Source: CAD feature listing. Evaluate the final solid. Frame: model axes, mm. Face numbers are marked on the shaded views. A direction names the side the tool comes from. Coordinates: 2 decimals unless noted, no trailing zeros. Loops run counter-clockwise (first coordinate to the right, second up) from the corner with the lowest first, then second, coordinate; pieces in that order, holes last. Notation, with made-up numbers: (3.25, 11) -> (15.25, 11) arc R12 ccw to (15.25, 30) -> close; hole circle Ø7 at (37, -33.75). An arc over 180 degrees is marked (long way). Answer as a JSON object with one key per item and string values. Group by question number.
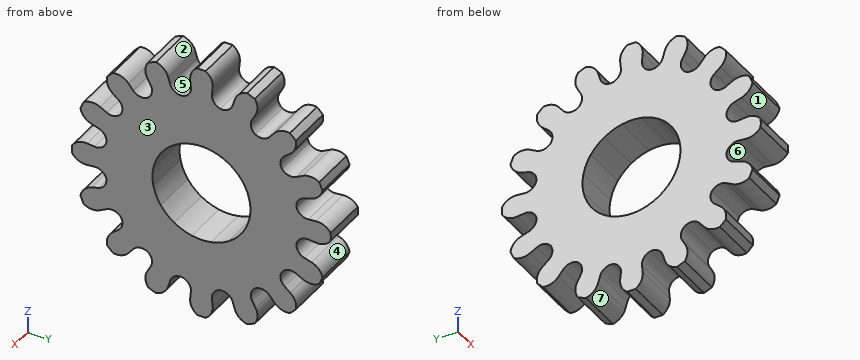
from build123d import *

# Parameters (mm, degrees)
BOSS_EXTRUDE2_DEPTH = 3.175
FILLET1_R           = 0.767540966
CIRPATTERN1_COUNT   = 16
SKETCH2_R           = 3.41
CUT_EXTRUDE1_DEPTH  = 14.117950488


with BuildPart() as part:
    # Sketch1 → Boss-Extrude2 (new body)
    with BuildSketch(Plane(origin=(0, 0, 0), x_dir=(0, 0, -1), z_dir=(1, 0, 0))):
        with BuildLine():
            Line((6.717496905, 0.661615697), (7.961477813, 0.784137123))
            ThreePointArc((7.961477813, 0.784137123), (8.546163052, 0.682503707), (8.995181287, 0.294471745))
            ThreePointArc((8.995181287, 0.294471745), (9, 0), (8.995181287, -0.294471745))
            ThreePointArc((8.995181287, -0.294471745), (8.546163052, -0.682503707), (7.961477813, -0.784137123))
            Line((7.961477813, -0.784137123), (6.717496905, -0.661615697))
            ThreePointArc((6.717496905, -0.661615697), (6.676941442, -0.990430703), (6.620300643, -1.316859674))
            Line((6.620300643, -1.316859674), (0, 0))
            Line((0, 0), (6.620300643, 1.316859674))
            ThreePointArc((6.620300643, 1.316859674), (6.676941442, 0.990430703), (6.717496905, 0.661615697))
        make_face()
    extrude(amount=BOSS_EXTRUDE2_DEPTH)

    # Fillet1
    # the kernel refuses this fillet: 0.767540966 mm, written as the material it adds along each edge
    with BuildSketch(Plane(origin=(0, 0.661615697, -6.717496905), x_dir=(0, 0.9888733768354266, 0.14875968736892464), z_dir=(1, 0, 0))) as fillet1_piece_1_section:
        with BuildLine():
            CenterArc((0.729311441, -0.766537545), FILLET1_R, 92.930055473, 84.139889054)
            Line((-0.037226104, -0.727303285), (0, 0))
            ThreePointArc((0, 0), (0.345038591, -0.008824407), (0.690077182, 0))
        make_face()
    fillet1_piece_1 = extrude(amount=3.175, mode=Mode.PRIVATE)
    fillet1_piece_1 = split(fillet1_piece_1, bisect_by=Plane(origin=(1.5875, 1.34516519, -6.762602082), z_dir=(0, -0.9807852804032304, -0.19509032201612872)), keep=Keep.TOP, mode=Mode.PRIVATE)
    add(fillet1_piece_1)
    with BuildSketch(Plane(origin=(0, -0.661615697, -6.717496905), x_dir=(0, -0.09801714032956141, -0.9951847266721968), z_dir=(1, 0, 0))) as fillet1_piece_2_section:
        with BuildLine():
            CenterArc((0.728255348, -0.767540966), FILLET1_R, 90, 84.139889054)
            ThreePointArc((-0.035274557, -0.68917503), (-0.008824407, -0.345038591), (0, 0))
            Line((0, 0), (0.728255348, 0))
        make_face()
    fillet1_piece_2 = extrude(amount=3.175, mode=Mode.PRIVATE)
    fillet1_piece_2 = split(fillet1_piece_2, bisect_by=Plane(origin=(1.5875, -1.34516519, -6.762602082), z_dir=(0, 0.9807852804032304, -0.19509032201612872)), keep=Keep.TOP, mode=Mode.PRIVATE)
    add(fillet1_piece_2)


with BuildPart() as cirpattern1_1:
    # CirPattern1: pattern copy
    add(part.part.rotate(Axis((0, 0, 0), (1, 0, 0)), 1 * 360 / CIRPATTERN1_COUNT))


with BuildPart() as cirpattern1_2:
    # CirPattern1: pattern copy
    add(part.part.rotate(Axis((0, 0, 0), (1, 0, 0)), 2 * 360 / CIRPATTERN1_COUNT))


with BuildPart() as cirpattern1_3:
    # CirPattern1: pattern copy
    add(part.part.rotate(Axis((0, 0, 0), (1, 0, 0)), 3 * 360 / CIRPATTERN1_COUNT))


with BuildPart() as cirpattern1_4:
    # CirPattern1: pattern copy
    add(part.part.rotate(Axis((0, 0, 0), (1, 0, 0)), 4 * 360 / CIRPATTERN1_COUNT))


with BuildPart() as cirpattern1_5:
    # CirPattern1: pattern copy
    add(part.part.rotate(Axis((0, 0, 0), (1, 0, 0)), 5 * 360 / CIRPATTERN1_COUNT))


with BuildPart() as cirpattern1_6:
    # CirPattern1: pattern copy
    add(part.part.rotate(Axis((0, 0, 0), (1, 0, 0)), 6 * 360 / CIRPATTERN1_COUNT))


with BuildPart() as cirpattern1_7:
    # CirPattern1: pattern copy
    add(part.part.rotate(Axis((0, 0, 0), (1, 0, 0)), 7 * 360 / CIRPATTERN1_COUNT))


with BuildPart() as cirpattern1_8:
    # CirPattern1: pattern copy
    add(part.part.rotate(Axis((0, 0, 0), (1, 0, 0)), 8 * 360 / CIRPATTERN1_COUNT))


with BuildPart() as cirpattern1_9:
    # CirPattern1: pattern copy
    add(part.part.rotate(Axis((0, 0, 0), (1, 0, 0)), 9 * 360 / CIRPATTERN1_COUNT))


with BuildPart() as cirpattern1_10:
    # CirPattern1: pattern copy
    add(part.part.rotate(Axis((0, 0, 0), (1, 0, 0)), 10 * 360 / CIRPATTERN1_COUNT))


with BuildPart() as cirpattern1_11:
    # CirPattern1: pattern copy
    add(part.part.rotate(Axis((0, 0, 0), (1, 0, 0)), 11 * 360 / CIRPATTERN1_COUNT))


with BuildPart() as cirpattern1_12:
    # CirPattern1: pattern copy
    add(part.part.rotate(Axis((0, 0, 0), (1, 0, 0)), 12 * 360 / CIRPATTERN1_COUNT))


with BuildPart() as cirpattern1_13:
    # CirPattern1: pattern copy
    add(part.part.rotate(Axis((0, 0, 0), (1, 0, 0)), 13 * 360 / CIRPATTERN1_COUNT))


with BuildPart() as cirpattern1_14:
    # CirPattern1: pattern copy
    add(part.part.rotate(Axis((0, 0, 0), (1, 0, 0)), 14 * 360 / CIRPATTERN1_COUNT))


with BuildPart() as cirpattern1_15:
    # CirPattern1: pattern copy
    add(part.part.rotate(Axis((0, 0, 0), (1, 0, 0)), 15 * 360 / CIRPATTERN1_COUNT))


with BuildPart() as cut_extrude1_tool:
    # Sketch2 → Cut-Extrude1 (new, through all)
    with BuildSketch(Plane(origin=(3.175, 0, 0), x_dir=(0, 0, -1), z_dir=(1, 0, 0))):
        Circle(SKETCH2_R)
    extrude(amount=-CUT_EXTRUDE1_DEPTH)


with BuildPart() as part_1:
    add(part.part)

    # Cut-Extrude1: cut by cut_extrude1_tool
    add(cut_extrude1_tool.part, mode=Mode.SUBTRACT)


with BuildPart() as cirpattern1_1_1:
    add(cirpattern1_1.part)

    # Cut-Extrude1: cut by cut_extrude1_tool
    add(cut_extrude1_tool.part, mode=Mode.SUBTRACT)


with BuildPart() as cirpattern1_2_1:
    add(cirpattern1_2.part)

    # Cut-Extrude1: cut by cut_extrude1_tool
    add(cut_extrude1_tool.part, mode=Mode.SUBTRACT)


with BuildPart() as cirpattern1_3_1:
    add(cirpattern1_3.part)

    # Cut-Extrude1: cut by cut_extrude1_tool
    add(cut_extrude1_tool.part, mode=Mode.SUBTRACT)


with BuildPart() as cirpattern1_4_1:
    add(cirpattern1_4.part)

    # Cut-Extrude1: cut by cut_extrude1_tool
    add(cut_extrude1_tool.part, mode=Mode.SUBTRACT)


with BuildPart() as cirpattern1_5_1:
    add(cirpattern1_5.part)

    # Cut-Extrude1: cut by cut_extrude1_tool
    add(cut_extrude1_tool.part, mode=Mode.SUBTRACT)


with BuildPart() as cirpattern1_6_1:
    add(cirpattern1_6.part)

    # Cut-Extrude1: cut by cut_extrude1_tool
    add(cut_extrude1_tool.part, mode=Mode.SUBTRACT)


with BuildPart() as cirpattern1_7_1:
    add(cirpattern1_7.part)

    # Cut-Extrude1: cut by cut_extrude1_tool
    add(cut_extrude1_tool.part, mode=Mode.SUBTRACT)


with BuildPart() as cirpattern1_8_1:
    add(cirpattern1_8.part)

    # Cut-Extrude1: cut by cut_extrude1_tool
    add(cut_extrude1_tool.part, mode=Mode.SUBTRACT)


with BuildPart() as cirpattern1_9_1:
    add(cirpattern1_9.part)

    # Cut-Extrude1: cut by cut_extrude1_tool
    add(cut_extrude1_tool.part, mode=Mode.SUBTRACT)


with BuildPart() as cirpattern1_10_1:
    add(cirpattern1_10.part)

    # Cut-Extrude1: cut by cut_extrude1_tool
    add(cut_extrude1_tool.part, mode=Mode.SUBTRACT)


with BuildPart() as cirpattern1_11_1:
    add(cirpattern1_11.part)

    # Cut-Extrude1: cut by cut_extrude1_tool
    add(cut_extrude1_tool.part, mode=Mode.SUBTRACT)


with BuildPart() as cirpattern1_12_1:
    add(cirpattern1_12.part)

    # Cut-Extrude1: cut by cut_extrude1_tool
    add(cut_extrude1_tool.part, mode=Mode.SUBTRACT)


with BuildPart() as cirpattern1_13_1:
    add(cirpattern1_13.part)

    # Cut-Extrude1: cut by cut_extrude1_tool
    add(cut_extrude1_tool.part, mode=Mode.SUBTRACT)


with BuildPart() as cirpattern1_14_1:
    add(cirpattern1_14.part)

    # Cut-Extrude1: cut by cut_extrude1_tool
    add(cut_extrude1_tool.part, mode=Mode.SUBTRACT)


with BuildPart() as cirpattern1_15_1:
    add(cirpattern1_15.part)

    # Cut-Extrude1: cut by cut_extrude1_tool
    add(cut_extrude1_tool.part, mode=Mode.SUBTRACT)


with BuildPart() as cirpattern1_13_2:
    add(cirpattern1_13_1.part)

    # Combine1: union CirPattern1_1, CirPattern1_14, CirPattern1_2, CirPattern1_15, CirPattern1_3, part, CirPattern1_4, CirPattern1_5, CirPattern1_6, CirPattern1_7, CirPattern1_8, CirPattern1_9, CirPattern1_10, CirPattern1_11, CirPattern1_12
    add(cirpattern1_1_1.part)
    add(cirpattern1_14_1.part)
    add(cirpattern1_2_1.part)
    add(cirpattern1_15_1.part)
    add(cirpattern1_3_1.part)
    add(part_1.part)
    add(cirpattern1_4_1.part)
    add(cirpattern1_5_1.part)
    add(cirpattern1_6_1.part)
    add(cirpattern1_7_1.part)
    add(cirpattern1_8_1.part)
    add(cirpattern1_9_1.part)
    add(cirpattern1_10_1.part)
    add(cirpattern1_11_1.part)
    add(cirpattern1_12_1.part)


solid = cirpattern1_13_2.part
1. Mould query, pull axis Y, two halves, no side actions, for the marked faces 1, 2, 3 and 4. Classes: pulls with the +Y half, pulls with the -Y half, needs draft (parallel to the pull), parting line crosses it, or undercut.
2. Section query B-B on y = 4.25. Return loops of the section in (x, z) (3 decimals), then the cut area to 3 significant figures.
3. Pin query (flat end, axial travel): pin 1 Ø1 at (x, y) = (2.5, -7) entering from -Z; pin 2 Ø2 at (y, z) = (0, 3) entering from +X (3 decimals). Return the tip coordinate at first contact, or that it passes through.
4. Ray query, L1, parallel to Y at x = 2.5, z = 0; L2, parallel to Y at x = 2.3, z = -6.25; L3, parallel to Z at x = 0.9, y = 7. Return the intervals inside material, ascending.
5. Reachability of the marked faces 5, 6 and 7 from +Z, -Z, +X, -X, +Y, -Y: full face, straight path, thin tool, end or side. Return the list, or none.
6. Section query A-A on z = 1. Return loops of the section in (x, y) (3 decimals), then the cut area to 3 significant figures.
Solved:
{
 "1": {"face 1": "pulls with the -Y half", "face 2": "undercut", "face 3": "needs draft", "face 4": "pulls with the +Y half"},
 "2": {"outline": "(0, -5.507) -> (3.175, -5.507) -> (3.175, 5.507) -> (0, 5.507) -> close", "area": "35.0 mm^2"},
 "3": {"pin 1": "z = -6.22", "pin 2": "x = 3.175"},
 "4": {"L1": "-9 to -3.41, 3.41 to 9", "L2": "-6.48 to -5.13, -3.43 to 3.43, 5.13 to 6.48", "L3": "-3.74 to -2.1, -0.82 to 0.82, 2.1 to 3.74"},
 "5": {"face 5": "+Z, +X, -X", "face 6": "+X, -X", "face 7": "-Z, +X, -X"},
 "6": {"outline": "(0, -6.782) -> (3.175, -6.782) -> (3.175, -3.26) -> (0, -3.26) -> close; (0, 3.26) -> (3.175, 3.26) -> (3.175, 6.782) -> (0, 6.782) -> close", "area": "22.4 mm^2"}
}
